from build123d import *

# Parameters (mm, degrees)
RESSALTO_EXTRUS_O1_DEPTH = 5
ESBO_O3_W                = 4
ESBO_O3_H                = 4
RESSALTO_EXTRUS_O2_DEPTH = 5
ESBO_O5_W                = 9.102985385
ESBO_O5_H                = 2
CORTE_EXTRUS_O1_DEPTH    = 5


with BuildPart() as part:
    # Esboço2 → Ressalto-extrusão1 (new body)
    with BuildSketch(Plane(origin=(0, 0, 0), x_dir=(1, 0, 0), z_dir=(0, 1, 0))):
        with BuildLine():
            ThreePointArc((-2.4, -5.499090834), (3.286335345, -5.019960159), (6, 0))
            Line((6, 0), (4, 0))
            ThreePointArc((4, 0), (0, -4), (-4, 0))
            Line((-4, 0), (-6, 0))
            ThreePointArc((-6, 0), (-5.019960159, -3.286335345), (-2.4, -5.499090834))
        make_face()
        with BuildLine():
            Line((4, 0), (6, 0))
            ThreePointArc((6, 0), (3.286335345, 5.019960159), (-2.4, 5.499090834))
            ThreePointArc((-2.4, 5.499090834), (-5.019960159, 3.286335345), (-6, 0))
            Line((-6, 0), (-4, 0))
            ThreePointArc((-4, 0), (0, 4), (4, 0))
        make_face()
        with BuildLine():
            Line((-10.8, -1.833030278), (-2.4, -5.499090834))
            ThreePointArc((-2.4, -5.499090834), (-5.019960159, -3.286335345), (-6, 0))
            Line((-6, 0), (-8, 0))
            ThreePointArc((-8, 0), (-8.904554885, -1.673320053), (-10.8, -1.833030278))
        make_face()
        with BuildLine():
            ThreePointArc((-6, 0), (-5.019960159, 3.286335345), (-2.4, 5.499090834))
            Line((-2.4, 5.499090834), (-10.8, 1.833030278))
            ThreePointArc((-10.8, 1.833030278), (-8.904554885, 1.673320053), (-8, 0))
            Line((-8, 0), (-6, 0))
        make_face()
        with BuildLine():
            ThreePointArc((-8, 0), (-8.904554885, 1.673320053), (-10.8, 1.833030278))
            ThreePointArc((-10.8, 1.833030278), (-11.673320053, 1.095445115), (-12, 0))
            Line((-12, 0), (-8, 0))
        make_face()
        with BuildLine():
            ThreePointArc((-12, 0), (-11.673320053, -1.095445115), (-10.8, -1.833030278))
            ThreePointArc((-10.8, -1.833030278), (-8.904554885, -1.673320053), (-8, 0))
            Line((-8, 0), (-12, 0))
        make_face()
    extrude(amount=RESSALTO_EXTRUS_O1_DEPTH)

    # Esboço3 → Ressalto-extrusão2 (add, through all)
    with BuildSketch(Plane(origin=(0, 5, 0), x_dir=(1, 0, 0), z_dir=(0, 1, 0))):
        with Locations((7.656854249, 0)):
            Rectangle(ESBO_O3_W, ESBO_O3_H)
    extrude(amount=-RESSALTO_EXTRUS_O2_DEPTH)

    # Esboço5 → Corte-extrusão1 (cut)
    with BuildSketch(Plane(origin=(0, 5, 0), x_dir=(1, 0, 0), z_dir=(0, 1, 0))):
        with Locations((6.873009698, 0)):
            Rectangle(ESBO_O5_W, ESBO_O5_H)
    extrude(amount=-CORTE_EXTRUS_O1_DEPTH, mode=Mode.SUBTRACT)


solid = part.part
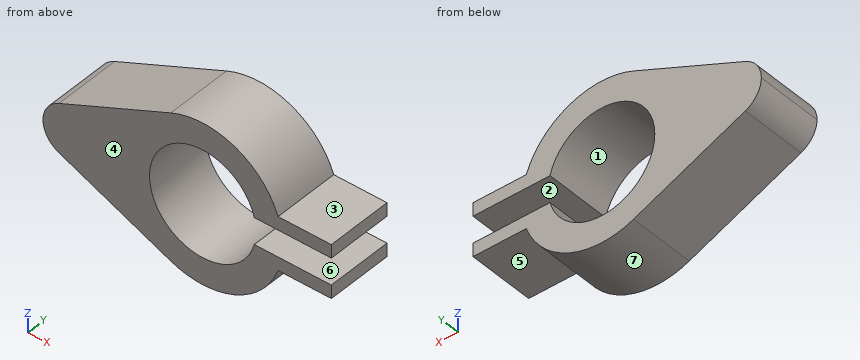
Geometry: final body of the model. Coordinates: model frame, mm. Face numbers are marked on the shaded views. A direction names the side the tool comes from. Give positions to 0.01 mm unless a question says otherwise; leave off trailing zeros. Write each loop counter-clockwise with the first axis right and the second up, starting at its lowest first coordinate (ties: lowest second). Pieces come first, ordered by that corner, then holes. Notation, with made-up numbers: M 69.5,66 L 118.5,66 A17 ccw 118.5,91 Z; hole C 8,48 d8. An arc over 180 degrees is marked long. Answer in a Markdown table with one row per item. Add a question column.
(1) Reachability of the marked faces 5, 6 and 7 from +Z, -Z, +X, -X, +Y, -Y: full face, straight path, thin tool, end or side. Return the list, or none.
(2) Section D-D on z = -0.75. Return loops of the section in (x, y), and give its area (3 significant figures).
(3) Section A-A on x = 0. Return loops of the section in (y, z).
(4) Section C-C on z = 2.5. Return loops of the section in (x, y).
(5) Mould query, pull axis Z, two halves, no side actions, for the marked faces 1, 2, 3 and 4. Classes: +Z half, -Z half, draft (parallel to the pull), parting line (faces both ways), or undercut.
(6) First-contact query: pin 1 (1.5 mm diameter, centred on y = 4, z = 1, fed in from -X); pin 2 (1.5 mm diameter, centred on y = 1.5, z = -4, fed in from +X); pin 3 (1.5 mm diameter, centred on x = -9, y = 1, fed in from +Z). Flat tips, straight axial feed; report the tip coordinate or a pass-through.
(7) Section B-B on y = 0.75. Return loops of the section in (x, z), and give its area (3 significant figures).
(8) Ray query, line 1 (Z direction, x = 0, y = 3.4); line 2 (X direction, y = 1.75, z = 3); line 3 (Z direction, x = 0.75, y = 2.8). Return the intervals inside material, ascending.
Result set:
| question | item | result |
|---|---|---|
| 1 | face 5 | -Z, +X, +Y, -Y |
| 1 | face 6 | +X, +Y, -Y |
| 1 | face 7 | -Z, +Y, -Y |
| 2 | outline | M -11.85,0 L -3.93,0 L -3.93,5 L -11.85,5 Z |
| 2 | area | 39.6 mm^2 |
| 3 | outline | M 0,-6 L 5,-6 L 5,-4 L 0,-4 Z; M 0,4 L 5,4 L 5,6 L 0,6 Z |
| 4 | outline | M -9.27,0 L -3.12,0 L -3.12,5 L -9.27,5 Z; M 3.12,0 L 5.45,0 L 5.45,5 L 3.12,5 Z |
| 5 | face 1 | undercut |
| 5 | face 2 | undercut |
| 5 | face 3 | +Z half |
| 5 | face 4 | draft |
| 6 | pin 1 | stops at x = -11.98 |
| 6 | pin 2 | stops at x = 5.04 |
| 6 | pin 3 | stops at z = 2.95 |
| 7 | outline | M -10.8,-1.83 L -2.4,-5.5 A6 ccw 5.66,-2 L 9.66,-2 L 9.66,-1 L 3.87,-1 A4 cw long 3.87,1 L 9.66,1 L 9.66,2 L 5.66,2 A6 ccw -2.4,5.5 L -10.8,1.83 A2 ccw Z |
| 7 | area | 103 mm^2 |
| 8 | line 1 | z = -6 to -4, 4 to 6 |
| 8 | line 2 | x = -8.13 to -2.65, 2.65 to 5.2 |
| 8 | line 3 | z = -5.95 to -3.93, 3.93 to 5.95 |
